from build123d import *

# Parameters (mm, degrees)
SKETCH1_R           = 13.5
SKETCH1_R_2         = 1.7
SKETCH1_R_3         = 5.5
BOSS_EXTRUDE1_DEPTH = 2.5
SKETCH2_R           = 13.5
SKETCH2_R_2         = 12.65
BOSS_EXTRUDE2_DEPTH = 3
SKETCH3_W           = 25
SKETCH3_H           = 25
SKETCH3_R           = 3
BOSS_EXTRUDE3_DEPTH = 4.5
CHAMFER2_SIZE       = 0.3
SKETCH4_R           = 4
BOSS_EXTRUDE4_DEPTH = 1.5
CUT_EXTRUDE1_DEPTH  = 20.868316486
CHAMFER3_SIZE       = 0.3
BOSS_EXTRUDE5_DEPTH = 4.5
CHAMFER4_SIZE       = 0.3
FILLET1_R           = 0.3
SKETCH8_R           = 1.5
CUT_EXTRUDE2_DEPTH  = 3
CHAMFER5_SIZE       = 2


with BuildPart() as part:
    # Sketch1 → Boss-Extrude1 (new body)
    with BuildSketch(Plane(origin=(0, 0, 0), x_dir=(1, 0, 0), z_dir=(0, 1, 0))):
        with Locations(Location((0, 0, 0), (0, 0, 270))):
            Circle(SKETCH1_R)
        with Locations(Location((6.646803743, 6.646803743, 0), (0, 0, 270))):
            Circle(SKETCH1_R_2, mode=Mode.SUBTRACT)
        with Locations(Location((-6.646803743, -6.646803743, 0), (0, 0, 270))):
            Circle(SKETCH1_R_2, mode=Mode.SUBTRACT)
        with Locations(Location((5.533110563, -5.533110563, 0), (0, 0, 270))):
            Circle(SKETCH1_R_2, mode=Mode.SUBTRACT)
        with Locations(Location((-5.533110563, 5.533110563, 0), (0, 0, 270))):
            Circle(SKETCH1_R_2, mode=Mode.SUBTRACT)
        with Locations(Location((0, 0, 0), (0, 0, 270))):
            Circle(SKETCH1_R_3, mode=Mode.SUBTRACT)
    extrude(amount=BOSS_EXTRUDE1_DEPTH)

    # Sketch2 → Boss-Extrude2 (add)
    with BuildSketch(Plane(origin=(0, 2.5, 0), x_dir=(1, 0, 0), z_dir=(0, 1, 0))):
        with Locations(Location((0, 0, 0), (0, 0, 270))):
            Circle(SKETCH2_R)
        with Locations(Location((0, 0, 0), (0, 0, 270))):
            Circle(SKETCH2_R_2, mode=Mode.SUBTRACT)
    extrude(amount=BOSS_EXTRUDE2_DEPTH)

    # Sketch3 → Boss-Extrude3 (add)
    with BuildSketch(Plane.XZ):
        Rectangle(SKETCH3_W, SKETCH3_H)
        with Locations(Location((-6.646803743, 6.646803743, 0), (0, 0, 270))):
            Circle(SKETCH3_R, mode=Mode.SUBTRACT)
        with Locations(Location((5.533110563, 5.533110563, 0), (0, 0, 193.381478788))):
            Circle(SKETCH3_R, mode=Mode.SUBTRACT)
        with Locations(Location((6.646803743, -6.646803743, 0), (0, 0, 270))):
            Circle(SKETCH3_R, mode=Mode.SUBTRACT)
        with Locations(Location((-5.533110563, -5.533110563, 0), (0, 0, 76.618521212))):
            Circle(SKETCH3_R, mode=Mode.SUBTRACT)
    extrude(amount=BOSS_EXTRUDE3_DEPTH)

    # Chamfer2
    chamfer2_edges = [part.edges().sort_by_distance(p)[0] for p in [
        (0, 2.5, -12.65),
    ]]
    chamfer(chamfer2_edges, length=CHAMFER2_SIZE)

    # Sketch4 → Boss-Extrude4 (add)
    # profile 1 of 3: a face of its own
    with BuildSketch(Plane(origin=(0, 0, 0), x_dir=(1, 0, 0), z_dir=(0, 1, 0))):
        with BuildLine():
            ThreePointArc((-4.838810256, 2.614558339), (-3.889087297, -3.889087297), (2.614558339, -4.838810256))
            ThreePointArc((2.614558339, -4.838810256), (3.411790219, -3.411790219), (4.838810256, -2.614558339))
            ThreePointArc((4.838810256, -2.614558339), (3.889087297, 3.889087297), (-2.614558339, 4.838810256))
            ThreePointArc((-2.614558339, 4.838810256), (-3.411790219, 3.411790219), (-4.838810256, 2.614558339))
        make_face()
        with Locations(Location((0, 0, 0), (0, 0, 270))):
            Circle(SKETCH4_R, mode=Mode.SUBTRACT)
    # profile 2 of 3: a face of its own
    with BuildSketch(Plane(origin=(0, 0, 0), x_dir=(1, 0, 0), z_dir=(0, 1, 0))):
        with BuildLine():
            ThreePointArc((-4.838810256, 2.614558339), (-3.411790219, 3.411790219), (-2.614558339, 4.838810256))
            ThreePointArc((-2.614558339, 4.838810256), (-3.889087297, 3.889087297), (-4.838810256, 2.614558339))
        make_face()
    # profile 3 of 3: a face of its own
    with BuildSketch(Plane(origin=(0, 0, 0), x_dir=(1, 0, 0), z_dir=(0, 1, 0))):
        with BuildLine():
            ThreePointArc((2.614558339, -4.838810256), (3.889087297, -3.889087297), (4.838810256, -2.614558339))
            ThreePointArc((4.838810256, -2.614558339), (3.411790219, -3.411790219), (2.614558339, -4.838810256))
        make_face()
    extrude(amount=BOSS_EXTRUDE4_DEPTH)

    # Sketch6 → Cut-Extrude1 (cut, through all)
    with BuildSketch(Plane.XZ):
        with BuildLine():
            Line((5.099019514, -12.5), (-5.099019514, -12.5))
            ThreePointArc((-5.099019514, -12.5), (0, -13.5), (5.099019514, -12.5))
        make_face()
        with BuildLine():
            Line((12.5, 5.099019514), (12.5, -5.099019514))
            ThreePointArc((12.5, -5.099019514), (13.5, 0), (12.5, 5.099019514))
        make_face()
        with BuildLine():
            Line((-5.099019514, 12.5), (5.099019514, 12.5))
            ThreePointArc((5.099019514, 12.5), (0, 13.5), (-5.099019514, 12.5))
        make_face()
        with BuildLine():
            Line((-12.5, -5.099019514), (-12.5, 5.099019514))
            ThreePointArc((-12.5, 5.099019514), (-13.5, 0), (-12.5, -5.099019514))
        make_face()
    extrude(amount=-CUT_EXTRUDE1_DEPTH, mode=Mode.SUBTRACT)

    # Chamfer3
    chamfer3_edges = [part.edges().sort_by_distance(p)[0] for p in [
        (8.944900782, 5.5, -8.944900782),
        (-8.944900782, 5.5, -8.944900782),
        (-8.944900782, 5.5, 8.944900782),
        (8.944900782, 5.5, 8.944900782),
    ]]
    chamfer(chamfer3_edges, length=CHAMFER3_SIZE)

    # Sketch7 → Boss-Extrude5 (add)
    with BuildSketch(Plane.XZ.offset(4.5)):
        Polygon((-12.5, 12.5), (-10, 12.5), (-10, 15.5), align=None)
        Polygon((-10, 12.5), (-7.5, 12.5), (-7.5, 15.5), align=None)
        Polygon((-7.5, 12.5), (-5, 12.5), (-5, 15.5), align=None)
        Polygon((-5, 12.5), (-2.5, 12.5), (-2.5, 15.5), align=None)
        Polygon((-2.5, 12.5), (0, 12.5), (0, 15.5), align=None)
        Polygon((0, 12.5), (2.5, 12.5), (2.5, 15.5), align=None)
        Polygon((2.5, 12.5), (5, 12.5), (5, 15.5), align=None)
        Polygon((5, 12.5), (7.5, 12.5), (7.5, 15.5), align=None)
        Polygon((7.5, 12.5), (10, 12.5), (10, 15.5), align=None)
        Polygon((10, 12.5), (12.5, 12.5), (12.5, 15.5), align=None)
    extrude(amount=-BOSS_EXTRUDE5_DEPTH)

    # Chamfer4
    chamfer4_edges = [part.edges().sort_by_distance(p)[0] for p in [
        (-11.25, -4.5, 14),
        (-10, -4.5, 14),
        (-7.5, -4.5, 14),
        (-8.75, -4.5, 14),
        (-5, -4.5, 14),
        (-6.25, -4.5, 14),
        (-2.5, -4.5, 14),
        (-3.75, -4.5, 14),
        (0, -4.5, 14),
        (-1.25, -4.5, 14),
        (2.5, -4.5, 14),
        (1.25, -4.5, 14),
        (5, -4.5, 14),
        (3.75, -4.5, 14),
        (7.5, -4.5, 14),
        (6.25, -4.5, 14),
        (10, -4.5, 14),
        (8.75, -4.5, 14),
        (11.25, -4.5, 14),
        (0, -4.5, -12.5),
    ]]
    chamfer(chamfer4_edges, length=CHAMFER4_SIZE)

    # Fillet1
    fillet1_edges = [part.edges().sort_by_distance(p)[0] for p in [
        (10, -2.1, 15.5),
        (7.5, -2.1, 15.5),
        (5, -2.1, 15.5),
        (2.5, -2.1, 15.5),
        (0, -2.1, 15.5),
        (-2.5, -2.1, 15.5),
        (-5, -2.1, 15.5),
        (-7.5, -2.1, 15.5),
        (-10, -2.1, 15.5),
        (12.5, -2.1, 15.5),
    ]]
    fillet(fillet1_edges, radius=FILLET1_R)

    # Sketch8 → Cut-Extrude2 (cut)
    with BuildSketch(Plane.XZ.offset(4.5)):
        with Locations(Location((0, 0, 0), (0, 0, 270))):
            Circle(SKETCH8_R)
    extrude(amount=-CUT_EXTRUDE2_DEPTH, mode=Mode.SUBTRACT)

    # Chamfer5
    # the kernel refuses this chamfer: 2 mm, written as the material it adds along each edge
    with BuildSketch(Plane(origin=(-5.533110563, 0, -5.533110563), x_dir=(0.2314334356248564, 0, 0.9728507413138335), z_dir=(0.9728507413138335, 0, -0.2314334356248564))) as chamfer5_piece_1_section:
        Polygon((3, CHAMFER5_SIZE), (3 - CHAMFER5_SIZE, 0), (3, 0), align=None)
    chamfer5_piece_1 = revolve(axis=Axis((-5.533110563, 0, -5.533110563), (0, -1, 0)), mode=Mode.PRIVATE)
    chamfer5_piece_1 = chamfer5_piece_1 - Plane(origin=(-5.533110563, -1.35638922, -5.533110563), x_dir=(0, 0, 1), z_dir=(0, -1, 0)) * Cylinder(1.7, 13, mode=Mode.PRIVATE)
    add(chamfer5_piece_1)
    with BuildSketch(Plane(origin=(5.533110563, 0, 5.533110563), x_dir=(-0.9728507413138336, 0, -0.23143343562485635), z_dir=(-0.23143343562485635, 0, 0.9728507413138336))) as chamfer5_piece_2_section:
        Polygon((3, CHAMFER5_SIZE), (3 - CHAMFER5_SIZE, 0), (3, 0), align=None)
    chamfer5_piece_2 = revolve(axis=Axis((5.533110563, 0, 5.533110563), (0, -1, 0)), mode=Mode.PRIVATE)
    chamfer5_piece_2 = chamfer5_piece_2 - Plane(origin=(5.533110563, -1.35638922, 5.533110563), x_dir=(0, 0, 1), z_dir=(0, -1, 0)) * Cylinder(1.7, 12, mode=Mode.PRIVATE)
    add(chamfer5_piece_2)
    with BuildSketch(Plane(origin=(6.646803743, 0, -6.646803743), x_dir=(0, 0, -1), z_dir=(-1, 0, 0))) as chamfer5_piece_3_section:
        Polygon((3, CHAMFER5_SIZE), (3 - CHAMFER5_SIZE, 0), (3, 0), align=None)
    chamfer5_piece_3 = revolve(axis=Axis((6.646803743, 0, -6.646803743), (0, -1, 0)), mode=Mode.PRIVATE)
    chamfer5_piece_3 = chamfer5_piece_3 - Plane(origin=(6.646803743, -1.35638922, -6.646803743), x_dir=(0, 0, 1), z_dir=(0, -1, 0)) * Cylinder(1.7, 13, mode=Mode.PRIVATE)
    add(chamfer5_piece_3)
    with BuildSketch(Plane(origin=(-6.646803743, 0, 6.646803743), x_dir=(0, 0, -1), z_dir=(-1, 0, 0))) as chamfer5_piece_4_section:
        Polygon((3, CHAMFER5_SIZE), (3 - CHAMFER5_SIZE, 0), (3, 0), align=None)
    chamfer5_piece_4 = revolve(axis=Axis((-6.646803743, 0, 6.646803743), (0, -1, 0)), mode=Mode.PRIVATE)
    chamfer5_piece_4 = chamfer5_piece_4 - Plane(origin=(-6.646803743, -1.35638922, 6.646803743), x_dir=(0, 0, 1), z_dir=(0, -1, 0)) * Cylinder(1.7, 13, mode=Mode.PRIVATE)
    add(chamfer5_piece_4)


solid = part.part
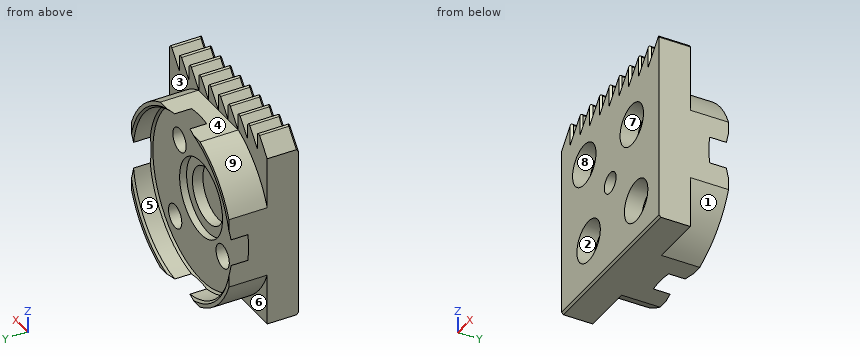
Can you work these out from the model? Positions are in its coordinate system, mm. Face numbers are marked on the shaded views. A direction names the side the tool comes from. Round coordinates to 2 decimals unless told otherwise and drop trailing zeros. Write each question's results on one line, items separated by ' | '. Start each with the question number.
1) For pin 1 Ø10.5 at (x, z) = (0, 0) entering from +Y; pin 2 Ø6.5 at (x, z) = (0, 0) entering from +Y; pin 3 Ø3 at (y, z) = (2.5, 9.5) entering from +X, each with a flat end and sliding along its axis, tell me the tip position at first contact or that it passes through.
2) Suppose I cut it at A-A (x = -6). Give the number of separate pieces and of enclosed holes in the cut face, and give its area (3 significant figures).
3) Please list where these lines run through material, in increasing order: line 1 (X direction, y = -3.5, z = 5.25); line 2 (X direction, y = -3.3, z = 0); line 3 (Z direction, x = 6, y = -4).
4) Which directions (+Z, -Z, +X, -X, +Y, -Y) give clear straight access to the entire face, cutting with the end or side of a thin tool? Please do the marked faces 1, 2, 3, 4 and 5.
5) We'd pull the mould along Z, two halves only. Please class the marked faces 6, 7, 8 and 9: released by +Z, released by -Z, zero draft, split by the parting line, or undercut.
Here are the results:
1) pin 1: stops at y = 1.5 | pin 2: stops at y = 0 | pin 3: stops at x = 10.87
2) separate pieces: 3 | enclosed holes: 0 | area: 125 mm2
3) line 1: x = -12.5 to -9.3, -3.99 to 2.55, 8.52 to 12.5 | line 2: x = -12.5 to -1.5, 1.5 to 12.5 | line 3: z = -12.5 to -9.58, -3.72 to 2.57, 8.5 to 13.7
4) face 1: -Z, +X, +Y | face 2: -Y | face 3: +Z, +X, +Y | face 4: +Z, +X, -X, +Y | face 5: +Y
5) face 6: zero draft | face 7: undercut | face 8: undercut | face 9: released by +Z
